Autodesk Inventor part; units mm, degrees
ref_plane "YZ Plane" through (0, 0, 0) normal (1, 0, 0) x (0, 1, 0)
ref_plane "XZ Plane" through (0, 0, 0) normal (0, 1, 0) x (-1, 0, 0)
ref_plane "XY Plane" through (0, 0, 0) normal (0, 0, 1) x (1, 0, 0)
sketch "Sketch1" plane through (0, 0, 0) normal (0, 1, 0) x (-1, 0, 0)
  line L0 (0, 0) -> (-384, 0)
  line L1 (-384, 0) -> (-384, -343)
  line L2 (-384, -343) -> (0, -343)
  line L3 (0, -343) -> (0, 0)
  dimension "d0" = 384
  dimension "d1" = 343
extrude "Extrusion1" add sketch "Sketch1" along normal blind 48.5
sketch "Sketch3" plane through (384, 0, 0) normal (1, 0, 0) x (0, 0, -1)
  line L0 (0, 0) -> (343, 0)
  line L1 (0, 0) -> (0, 48.5)
  line L2 (343, 0) -> (343, 48.5)
  line L3 (30, 48.5) -> (65, 48.5)
  line L4 (30, 48.5) -> (30, 37)
  line L5 (65, 48.5) -> (74.6496, 37)
  line L6 (43, 37) -> (74.6496, 37)
  line L7 (30, 37) -> (30, 35)
  line L8 (30, 35) -> (43, 35)
  line L9 (43, 35) -> (43, 37)
  dimension "d23" = 35
  dimension "d37" = 2
  dimension "d38" = 13
extrude "Extrusion2" cut sketch "Sketch3" against normal through all
sketch "Sketch7" plane through (384, 0, 0) normal (1, 0, 0) x (0, 0, -1)
  line L0 (65, 48.5) -> (343, 48.5)
  line L1 (65, 48.5) -> (161, 48.5)
  line L2 (161, 48.5) -> (174.2196, 48.5) construction
  line L3 (161, 48.5) -> (205, 48.5)
  line L4 (0, 0) -> (343, 0)
  line L5 (151.3504, 37) -> (192, 37)
  line L6 (205, 37) -> (205, 48.5)
  line L7 (161, 48.5) -> (151.3504, 37)
  line L8 (161, 48.5) -> (183.0653, 48.5) construction
  line L9 (205, 37) -> (205, 35)
  line L10 (205, 35) -> (192, 35)
  line L11 (192, 35) -> (192, 37)
  dimension "d27" = 96
  dimension "d29" = 44
  dimension "d32" = 130
extrude "Extrusion3" cut sketch "Sketch7" against normal through all
sketch "Sketch8" plane through (0, 48.5, 0) normal (0, 1, 0) x (1, 0, 0)
  line L0 (310, 343) -> (310, 316)
  line L1 (313, 313) -> (384, 313)
  line L2 (384, 0) -> (384, 343)
  line L3 (384, 313) -> (384, 343)
  line L4 (384, 343) -> (310, 343)
  line L5 (384, 343) -> (0, 343)
  arc A0 (310, 316) -> (313, 313) centre (313, 316) ccw
  point P0 (0, 0)
  point P1 (310, 313)
  dimension "d43" = 30
  dimension "d46" = 3
extrude "Extrusion4" cut sketch "Sketch8" against normal through all
sketch "Sketch12" plane through (0, 48.5, 0) normal (0, 1, 0) x (1, 0, 0)
  line L0 (221, 113) -> (221, 128)
  line L1 (211, 88) -> (0, 88)
  line L2 (211, 138) -> (0, 138)
  arc A0 (211, 88) -> (221, 98) centre (211, 98) ccw
  arc A1 (221, 128) -> (211, 138) centre (211, 128) ccw
  line L3 (221, 98) -> (221, 113)
  line L4 (0, 88) -> (0, 138)
  point P0 (384, 161)
  point P1 (221, 88)
  dimension "d72" = 10
extrude "Extrusion8" cut sketch "Sketch12" against normal blind 33
sketch "Sketch28" plane through (0, 48.5, 0) normal (0, 1, 0) x (1, 0, 0)
  circle A0 centre (373, 302) radius 5.8
  circle A1 centre (303.4, 302) radius 5.8
  circle A2 centre (373, 11) radius 5.8
  circle A3 centre (303.4, 11) radius 5.8
  point P0 (0, 0)
  point P1 (384, 313)
  point P2 (384, 0)
  dimension "d146" = 11.6
  dimension "d149" = 11.6
  dimension "d152" = 11.6
  dimension "d155" = 11.6
extrude "Extrusion19" cut sketch "Sketch28" against normal through all
sketch "Sketch30" plane through (0, 0, 0) normal (0, 0, 1) x (1, 0, 0)
  line L0 (48, 48.5) -> (215, 48.5)
  line L1 (215, 48.5) -> (215, 0)
  line L2 (215, 0) -> (48, 0)
  line L3 (48, 0) -> (48, 48.5)
  line L4 (0, 0) -> (0, 48.5)
  dimension "d255" = 48
  dimension "d256" = 167
extrude "Extrusion21" cut sketch "Sketch30" against normal up to surface (30 mm away)
sketch "Sketch32" plane through (0, 48.5, 0) normal (0, 1, 0) x (1, 0, 0)
  line L0 (275, 266) -> (283, 266) construction
  circle A0 centre (280.6569, 260.3431) radius 8
  point P0 (0, 0)
  point P1 (255, 343)
  dimension "d168" = 16
extrude "Extrusion22" cut sketch "Sketch32" against normal blind 10
sketch "Sketch36" plane through (0, 0, -343) normal (0, 0, -1) x (-1, 0, 0)
  line L0 (-255, 0) -> (-243.6863, 11.3137)
  line L1 (-255, 0) -> (-239, 0) construction
  line L2 (-243.6863, 11.3137) -> (-239.0863, 11.3137)
  line L3 (-239.0863, 11.3137) -> (-229.7525, 1.9799)
  line L4 (-239.0863, 11.3137) -> (-225.8863, 11.3137) construction
  line L5 (-229.7525, 1.9799) -> (-217.7525, 1.9799)
  line L6 (-22, 0) -> (-22, 10)
  line L7 (-22, 10) -> (-55, 10)
  line L8 (-217.7525, 1.9799) -> (-217.7525, 0)
  line L9 (-55, 10) -> (-55, 0)
  line L10 (-255, 0) -> (-217.7525, 0)
  line L11 (-310, 0) -> (0, 0)
  line L12 (-55, 0) -> (-22, 0)
  dimension "d209" = 16
  dimension "d210" = 45
  dimension "d211" = 4.6
  dimension "d214" = 13.2
  dimension "d215" = 45
  dimension "d216" = 12
  dimension "d224" = 22
  dimension "d225" = 10
extrude "Extrusion23" cut sketch "Sketch36" against normal through all
sketch "Sketch37" plane through (0, 0, -343) normal (0, 0, -1) x (-1, 0, 0)
  line L0 (-217.7525, 1.9799) -> (-217.7525, 15.9799)
  line L1 (-217.7525, 15.9799) -> (-241.3863, 48.5)
  line L2 (-241.3863, 48.5) -> (-19.5919, 48.5)
  line L3 (-211, 48.5) -> (0, 48.5)
  line L4 (-48, 10) -> (-55, 10)
  line L5 (-217.7525, 0) -> (-217.7525, 1.9799)
  line L6 (-217.7525, 1.9799) -> (-217.7525, 0)
  line L7 (-215, 0) -> (-55, 0)
  line L8 (-217.7525, 0) -> (-55, 0)
  line L9 (-55, 10) -> (-55, 0)
  line L10 (-55, 0) -> (-55, 10)
  line L11 (-217.7525, 15.9799) -> (-49.7525, 15.9799) construction
  line L12 (-55, 10) -> (-49.7525, 10)
  line L13 (-49.7525, 10) -> (-49.7525, 29)
  line L14 (-49.7525, 29) -> (-19.5919, 48.5)
  line L15 (0, 48.5) -> (-48, 48.5)
  point P0 (0, 0)
  point P1 (-23, 48.5)
  dimension "d229" = 14
  dimension "d232" = 19
extrude "Extrusion24" cut sketch "Sketch37" against normal blind 140
sketch "Sketch38" plane through (0, 0, -203) normal (0, 0, -1) x (-1, 0, 0)
  line L0 (-49.7525, 29) -> (-49.7525, 10)
  line L1 (-55, 9.9841) -> (-217.7525, 9.4921)
  line L2 (-217.7525, 1.9799) -> (-217.7525, 15.9799)
  line L3 (-217.7525, 0) -> (-217.7525, 1.9799)
  line L4 (-217.7525, 9.4921) -> (-217.7525, 0)
  line L5 (-215, 0) -> (-55, 0)
  line L6 (-217.7525, 0) -> (-55, 0)
  line L7 (-55, 10) -> (-55, 0)
  line L8 (-55, 0) -> (-55, 10)
  line L9 (-55, 10) -> (-55, 0)
  point P0 (0, 0)
extrude "Extrusion25" cut sketch "Sketch38" against normal through all
sketch "Sketch40" plane through (0, 0, -343) normal (0, 0, -1) x (-1, 0, 0)
  line L0 (-229.5482, 9.4921) -> (-238.1559, 19.4995)
  line L1 (-229.5482, 9.4921) -> (-216.3482, 9.4921) construction
  line L2 (-238.1559, 19.4995) -> (-242.7559, 19.4995)
  line L3 (-242.7559, 19.4995) -> (-255, 9.1999)
  line L4 (-242.7559, 19.4995) -> (-226.7559, 19.4995) construction
  line L5 (-243.6863, 11.3137) -> (-255, 0)
  line L6 (-255, 9.1999) -> (-255, 0)
  line L7 (-229.5482, 9.4921) -> (-217.7525, 9.4921)
  line L8 (-217.7525, 9.4921) -> (-217.7525, 1.9799)
  line L9 (-217.7525, 9.4921) -> (-217.7525, 1.9799)
  line L10 (-217.7525, 1.9799) -> (-217.7525, 9.4921)
  line L11 (-217.7525, 1.9799) -> (-229.7525, 1.9799)
  line L12 (-229.7525, 1.9799) -> (-239.0863, 11.3137)
  line L13 (-229.7525, 1.9799) -> (-239.0863, 11.3137)
  line L14 (-239.0863, 11.3137) -> (-243.6863, 11.3137)
  line L15 (-255, 0) -> (-243.6863, 11.3137)
  dimension "d240" = 13.2
  dimension "d242" = 4.6
  dimension "d243" = 16
extrude "Extrusion26" cut sketch "Sketch40" against normal through all
sketch "Sketch41" plane through (221, 48.5, -128) normal (-1, 0, 0) x (0, 0, 1)
  circle A0 centre (15, -16.5) radius 8.5
  point P0 (128, -48.5)
  dimension "d247" = 17
extrude "Extrusion27" cut sketch "Sketch41" against normal through all
sketch "Sketch42" plane through (384, 0, 0) normal (1, 0, 0) x (0, 0, -1)
  circle A0 centre (113, 32) radius 8.5
  circle A1 centre (113, 32) radius 14.5
  point P0 (0, 0)
  dimension "d250" = 29
extrude "Extrusion28" cut sketch "Sketch42" against normal blind 57
properties part number "saddle" material "Iron, Cast"
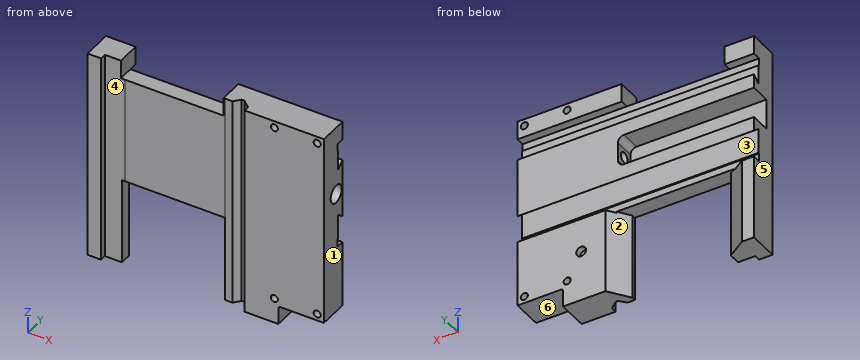
Geometry: final body of the model. Coordinates: model frame, mm. Face numbers are marked on the shaded views. A direction names the side the tool comes from. Give positions to 0.01 mm unless a question says otherwise; leave off trailing zeros. Order: outer loops, then holes, each group sorted by start corner. A loop starts at its lowest first (then second) coordinate and runs counter-clockwise, first axis right, second up. Notation, with made-up numbers: (31, 61) -> (54, 61) arc R20 cw to (54, 69) -> close; hole circle Ø7 at (80, 57.5). An arc over 180 degrees is marked (long way). Answer as a JSON object with one key per item and string values.
Q1. Draft query along X for the marked faces 4, 5 and 6. Return one class per face: released by +X, released by -X, zero draft, split by the parting line, or undercut.
Entries:
{"face 4": "undercut", "face 5": "released by -X", "face 6": "zero draft"}
Q2. Access query for the marked faces 1, 2 and 3. Directions: +Z, -Z, +X, -X, +Y, -Y. A direction counts if a zero-diameter tool reaches every point of the face in a straight line with its end or side. Return the directions, or none.
Entries:
{"face 1": "+Z, -Z, +X, +Y, -Y", "face 2": "-Z, +Y", "face 3": "+X, -X"}
Q3. Material intervals for probe 1 along Z at (x, y) = (303.4, 15); probe 2 along Z at (x, y) = (373, 14); probe 3 along X at (y, z) = (14, -26), sorted ascending.
Entries:
{"probe 1": "z = -343 to -307.8, -296.2 to -16.8, -5.2 to 0", "probe 2": "z = -313 to -307.8, -296.2 to -16.8, -5.2 to 0", "probe 3": "x = 0 to 48, 215 to 233.43, 249.29 to 384"}
Q4. Section C-C (z = -302). Output: boundary loops of the cut face in (x, y), plus the area to 3 significant figures.
Entries:
{"outline": "(0, 0) -> (22, 0) -> (22, 10) -> (49.75, 10) -> (49.75, 29) -> (19.59, 48.5) -> (0, 48.5) -> close; (217.75, 9.49) -> (229.55, 9.49) -> (238.16, 19.5) -> (242.76, 19.5) -> (255, 9.2) -> (255, 0) -> (297.6, 0) -> (297.6, 48.5) -> (241.39, 48.5) -> (217.75, 15.98) -> close; (309.2, 0) -> (367.2, 0) -> (367.2, 48.5) -> (309.2, 48.5) -> close; (378.8, 0) -> (384, 0) -> (384, 48.5) -> (378.8, 48.5) -> close", "area": "7,890 mm^2"}
Q5. Section D-D (x = 303.4). Output: boundary loops of the cut face in (y, z).
Entries:
{"outline": "(0, -343) -> (48.5, -343) -> (48.5, -307.8) -> (0, -307.8) -> close; (0, -296.2) -> (48.5, -296.2) -> (48.5, -205) -> (35, -205) -> (35, -192) -> (37, -192) -> (37, -151.35) -> (48.5, -161) -> (48.5, -65) -> (37, -74.65) -> (37, -43) -> (35, -43) -> (35, -30) -> (48.5, -30) -> (48.5, -16.8) -> (0, -16.8) -> close; (0, -5.2) -> (48.5, -5.2) -> (48.5, 0) -> (0, 0) -> close; hole circle Ø17 at (32, -113)"}
Q6. Section B-B (x = 373). Output: boundary loops of the cut face in (y, z), plus the area to 3 significant figures.
Entries:
{"outline": "(0, -313) -> (48.5, -313) -> (48.5, -307.8) -> (0, -307.8) -> close; (0, -296.2) -> (48.5, -296.2) -> (48.5, -205) -> (35, -205) -> (35, -192) -> (37, -192) -> (37, -151.35) -> (48.5, -161) -> (48.5, -65) -> (37, -74.65) -> (37, -43) -> (35, -43) -> (35, -30) -> (48.5, -30) -> (48.5, -16.8) -> (0, -16.8) -> close; (0, -5.2) -> (48.5, -5.2) -> (48.5, 0) -> (0, 0) -> close; hole circle Ø29 at (32, -113)", "area": "12,300 mm^2"}
Q7. First-contact query: pin 1 (9 mm diameter, centred on y = 37, z = -106, fed in from -X); pin 2 (1.5 mm diameter, centred on x = 326.5, z = -40.5, fed in from +Y); pin 3 (1 mm diameter, centred on x = 161.5, z = -99, fed in from -Y). Flat tips, straight axial feed; report the tip coordinate or a pass-through.
Entries:
{"pin 1": "stops at x = 221", "pin 2": "stops at y = 35", "pin 3": "stops at y = 9.66"}
